Part model, mm, in its own coordinate system. Face numbers are marked on the shaded views. A direction names the side the tool comes from. Coordinates: 2 decimals unless noted, no trailing zeros. Write each loop counter-clockwise with the first axis right and the second up, starting at its lowest first coordinate (ties: lowest second). Pieces come first, ordered by that corner, then holes. Notation, with made-up numbers: (-13, 62) -> (28, 62) arc R22 cw to (28, 85) -> close; hole circle Ø2 at (-7.75, 50.25). An arc over 180 degrees is marked (long way). Write item = value, one per line. Start each with the question number.
Q1. Pull direction X, two halves, no side cores. Call the marked faces 3, 4, 5 and 6: released by +X, released by -X, zero draft, split by the parting line, or undercut.
Q2. Band-saw the part on B-B, the plane y = 0. List the corners of the cut face in (x, z).
Q3. Pin check, flat tips, straight feed: P1, Ø4, axis at x = -145.5, z = 263.5, coming from the +Y side; P2, Ø15, axis at x = 103.5, z = 54.5, coming from the -Y side; P3, Ø10, axis at x = 148.5, z = 245, coming from the -Y side; P4, Ø6, axis at x = 6.5, y = -121.5, coming from the +Z side. Stop position of each tip, or through.
Q4. Band-saw the part on A-A, the plane z = 186. List the corners of the cut face in (x, y), plus the area to 3 significant figures.
Q5. Probe line 1 (Y direction, x = 114.3, z = 9.5) (3 decimals); line 2 (X direction, y = 114, z = 7); line 3 (X direction, y = 19, z = 45.5). List the from-to ranges inside material, lowest first.
Q6. Tool access for the marked faces 1 and 2: list every direction of +Z, -Z, +X, -X, +Y, -Y with a clear straight run to the whole face (end or side of a thin tool).
Q7. Band-saw the part on D-D, the plane y = -53.5. List the corners of the cut face in (x, z).
Q8. Band-saw the part on C-C, the plane x = 114.3. List the corners of the cut face in (y, z) (3 decimals), plus the area to 3 significant figures.
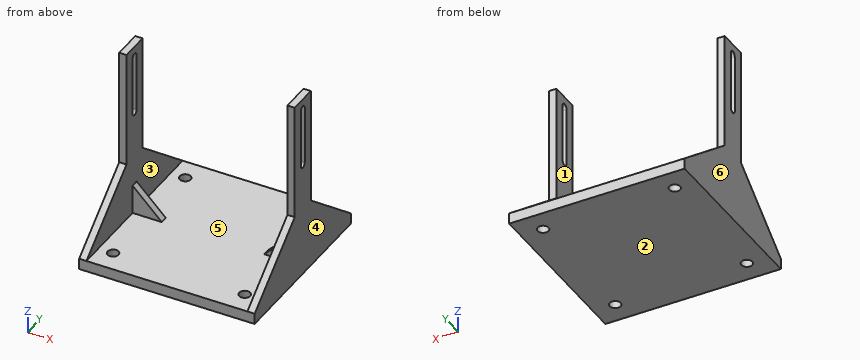
from build123d import *

# Parameters (mm, degrees)
F0_W      = 304.8
F0_H      = 304.8
F1_DEPTH  = 19.05
F2_W      = 12.7
F2_H      = 50.8
F3_DEPTH  = 304.8
F5_DEPTH  = 25.4
F7_DEPTH  = 6.35
F9_DEPTH  = 12.7
F10_R     = 9.525
F11_DEPTH = 25.4


# Not quite as in the source:
# - a pattern or mirror of a feature is missing from the dataset's text; its kind, count and spacing are read off the source's solid


with BuildPart() as f1:
    # F0 (on Top) → F1 (new body)
    with BuildSketch(Plane.XY):
        Rectangle(F0_W, F0_H)
    extrude(amount=F1_DEPTH)

    # F2 (on face) → F3 (join)
    with BuildSketch(Plane.XY.offset(19.05)):
        with Locations((146.05, 0)):
            Rectangle(F2_W, F2_H)
    f3 = extrude(amount=F3_DEPTH)

    # F3_copies: F3 across plane
    add(f3.mirror(Plane(origin=(0, 0, 0), x_dir=(0, 0, -1), z_dir=(-1, 0, 0))))

    # F4 (on face) → F5 (cut)
    with BuildSketch(Plane.YZ.offset(152.4)):
        with BuildLine():
            Line((6.35, 203.2), (6.35, 304.8))
            ThreePointArc((6.35, 304.8), (0, 311.15), (-6.35, 304.8))
            Line((-6.35, 304.8), (-6.35, 203.2))
            ThreePointArc((-6.35, 203.2), (0, 196.85), (6.35, 203.2))
        make_face()
    f5 = extrude(amount=-F5_DEPTH, mode=Mode.SUBTRACT)

    # F5_copies: F5 across plane
    add(f5.mirror(Plane(origin=(0, 0, 0), x_dir=(0, 0, -1), z_dir=(-1, 0, 0))), mode=Mode.SUBTRACT)

    # F6 (on Front) → F7 (join, symmetric)
    with BuildSketch(Plane.XZ):
        Polygon((139.7, 19.05), (139.7, 69.85), (88.9, 19.05), align=None)
    f7 = extrude(amount=F7_DEPTH, both=True)

    # F7_copies: F7 across plane
    add(f7.mirror(Plane(origin=(0, 0, 0), x_dir=(0, 0, -1), z_dir=(-1, 0, 0))))

    # F8 (on face) → F9 (join)
    with BuildSketch(Plane.YZ.offset(152.4)):
        Polygon((-25.4, 120.65), (-152.4, 19.05), (-25.4, 19.05), align=None)
        Polygon((152.4, 19.05), (25.4, 120.65), (25.4, 19.05), align=None)
    f9 = extrude(amount=-F9_DEPTH)

    # F9_copies: F9 across plane
    add(f9.mirror(Plane(origin=(0, 0, 0), x_dir=(0, 0, -1), z_dir=(-1, 0, 0))))

    # F10 (on face) → F11 (cut)
    with BuildSketch(Plane.XY.offset(19.05)):
        with Locations((-114.3, 114.3)):
            Circle(F10_R)
        with Locations((114.3, 114.3)):
            Circle(F10_R)
        with Locations((114.3, -114.3)):
            Circle(F10_R)
        with Locations((-114.3, -114.3)):
            Circle(F10_R)
    extrude(amount=-F11_DEPTH, mode=Mode.SUBTRACT)


solid = f1.part
Ans:
q1.face_3 = undercut
q1.face_4 = released by +X
q1.face_5 = undercut
q1.face_6 = released by -X
q2.outline = (-152.4, 0) -> (152.4, 0) -> (152.4, 196.85) -> (139.7, 196.85) -> (139.7, 69.85) -> (88.9, 19.05) -> (-88.9, 19.05) -> (-139.7, 69.85) -> (-139.7, 196.85) -> (-152.4, 196.85) -> close; (-152.4, 311.15) -> (-139.7, 311.15) -> (-139.7, 323.85) -> (-152.4, 323.85) -> close; (139.7, 311.15) -> (152.4, 311.15) -> (152.4, 323.85) -> (139.7, 323.85) -> close
q3.P1 = 25.4
q3.P2 = through
q3.P3 = -25.4
q3.P4 = 19.05
q4.outline = (-152.4, -25.4) -> (-139.7, -25.4) -> (-139.7, 25.4) -> (-152.4, 25.4) -> close; (139.7, -25.4) -> (152.4, -25.4) -> (152.4, 25.4) -> (139.7, 25.4) -> close
q4.area = 1,290 mm2
q5.line_1 = -152.4 to -123.825, -104.775 to 104.775, 123.825 to 152.4
q5.line_2 = -152.4 to -123.82, -104.78 to 104.78, 123.82 to 152.4
q5.line_3 = -152.4 to -139.7, 139.7 to 152.4
q6.face_1 = +Z
q6.face_2 = -Z, +X, -X, +Y, -Y
q7.outline = (-152.4, 0) -> (152.4, 0) -> (152.4, 98.17) -> (139.7, 98.17) -> (139.7, 19.05) -> (-139.7, 19.05) -> (-139.7, 98.17) -> (-152.4, 98.17) -> close
q8.outline = (-152.4, 0) -> (-123.825, 0) -> (-123.825, 19.05) -> (-152.4, 19.05) -> close; (-104.775, 0) -> (104.775, 0) -> (104.775, 19.05) -> (6.35, 19.05) -> (6.35, 44.45) -> (-6.35, 44.45) -> (-6.35, 19.05) -> (-104.775, 19.05) -> close; (123.825, 0) -> (152.4, 0) -> (152.4, 19.05) -> (123.825, 19.05) -> close
q8.area = 5,400 mm2
